Geometry check sheet. Reference: the model listing, model coordinates, mm. A direction names the side the tool comes from. Round coordinates to 2 decimals unless told otherwise and drop trailing zeros. Loops run counter-clockwise (first coordinate to the right, second up) from the corner with the lowest first, then second, coordinate; pieces in that order, holes last. Notation, with made-up numbers: (-36.75, -23) -> (-31.75, -23) arc R17 cw to (-31.75, 10) -> close; hole circle Ø1 at (59, 87.5). An arc over 180 degrees is marked (long way). Use a Markdown table: item, result. Add a question column.
Q1. Gauge pin test, flat ends, axial feed: P1, Ø4, axis at x = -0.5, z = 0, coming from the +Y side; P2, Ø1.5, axis at x = 3.5, z = 3.5, coming from the -Y side; P3, Ø3, axis at x = -0.5, y = 32.5, coming from the -Z side; P4, Ø1, axis at y = 12.5, z = -1, coming from the +X side. Record the tip position at first contact, or that the pin passes through.
Q2. Release check for a two-part mould opening along Z. For faces 4 (the face through (0, 0, 0)), 5 (the face through (0.67, 22.3, -3.04)), 6 (the face through (2.05, 48.92, 1.21)) record: released by +Z, released by -Z, zero draft, split by the parting line, or undercut.
Q3. Sectioned sample at B-B, the plane y = 36. Enter the section's corners in (x, z), then the cut area to 3 significant figures.
Q4. Material ranges on L1, parallel to Y at x = 3, z = -2.5; L2, parallel to Y at x = -2, z = 0; L3, parallel to X at y = 48.5, z = 2.25, recorded low to high.
Q5. Set-up check for faces 1 (the face through (-2.05, 48.92, -1.21)), 2 (the face through (-3, 44.45, -2)), 3 (the face through (0.61, 47.59, 4.66)): record each of +Z, -Z, +X, -X, +Y, -Y from which the full face is reachable in a straight line by a thin tool's end or side.
Q6. Sectioned sample at A-A, the plane x = 0. Enter the section's corners in (y, z), then the cut area to 3 significant figures.
```python
from build123d import *

# Parameters (mm, degrees)
EXTRUDE1_DEPTH = 3.81
FILLET1_R      = 0.381
CHAMFER1_SIZE  = 0.762


with BuildPart() as part:
    # Sketch1 → Revolve1 (revolve)
    with BuildSketch(Plane.XY):
        Polygon((0, 0), (0, 50.8), (-4.699, 50.8), (-4.699, 44.45), (-3.1115, 44.45), (-3.1115, 0), align=None)
    revolve(axis=Axis((0, 0, 0), (0, 1, 0)))

    # Sketch2 → Extrude1 (cut)
    with BuildSketch(Plane(origin=(0, 50.8, 0), x_dir=(1, 0, 0), z_dir=(0, 1, 0))):
        Polygon((2.7496262, 0), (1.3748131, 2.38124614), (-1.3748131, 2.38124614), (-2.7496262, 0), (-1.3748131, -2.38124614), (1.3748131, -2.38124614), align=None)
    extrude(amount=-EXTRUDE1_DEPTH, mode=Mode.SUBTRACT)

    # Fillet1
    fillet1_edges = [part.edges().sort_by_distance(p)[0] for p in [
        (4.699, 44.45, 0),
        (4.699, 50.8, 0),
    ]]
    fillet(fillet1_edges, radius=FILLET1_R)

    # Chamfer1
    chamfer1_edges = [part.edges().sort_by_distance(p)[0] for p in [
        (3.1115, 0, 0),
    ]]
    chamfer(chamfer1_edges, length=CHAMFER1_SIZE)


solid = part.part
```
Values:
| question | item | result |
|---|---|---|
| 1 | P1 | y = 50.8 |
| 1 | P2 | y = 44.45 |
| 1 | P3 | z = -3.11 |
| 1 | P4 | x = 3.07 |
| 2 | face 4 | zero draft |
| 2 | face 5 | split by the parting line |
| 2 | face 6 | undercut |
| 3 | outline | circle Ø6.22 at (0, 0) |
| 3 | area | 30.4 mm^2 |
| 4 | L1 | 44.45 to 50.8 |
| 4 | L2 | 0 to 46.99 |
| 4 | L3 | -4.13 to -1.45, 1.45 to 4.13 |
| 5 | face 1 | +Y |
| 5 | face 2 | -Y |
| 5 | face 3 | +Y, -Y |
| 6 | outline | (0, -2.35) -> (0.76, -3.11) -> (44.45, -3.11) -> (44.45, -4.32) arc R0.38 ccw to (44.83, -4.7) -> (50.42, -4.7) arc R0.38 ccw to (50.8, -4.32) -> (50.8, -2.38) -> (46.99, -2.38) -> (46.99, 2.38) -> (50.8, 2.38) -> (50.8, 4.32) arc R0.38 ccw to (50.42, 4.7) -> (44.83, 4.7) arc R0.38 ccw to (44.45, 4.32) -> (44.45, 3.11) -> (0.76, 3.11) -> (0, 2.35) -> close |
| 6 | area | 317 mm^2 |
